```python
from build123d import *

# Parameters (mm, degrees)
EXTRUDE_1_DEPTH        = 196
CUT_EXTRUDE_1_DEPTH    = 240.62524927
SKETCH_4_W             = 106
SKETCH_4_H             = 19
CUT_EXTRUDE_2_DEPTH    = 242.065053461
SKETCH_6_W             = 106
SKETCH_6_H             = 129
CUT_EXTRUDE_3_DEPTH    = 242.065053461
SKETCH_7_W             = 20
SKETCH_7_H             = 5
EXTRUDE_3_DEPTH        = 15
PATTERN_LINEAR_1_COUNT = 2
PATTERN_LINEAR_1_PITCH = 60
CUT_EXTRUDE_6_REACH    = 244.147
SKETCH_10_W            = 182
SKETCH_10_H            = 30.218365382
CUT_EXTRUDE_7_REACH    = 254.973
SKETCH_12_W            = 180
SKETCH_12_H            = 40.166727714
CUT_EXTRUDE_8_REACH    = 254.973
SKETCH_13_W            = 129
SKETCH_13_H            = 8
SKETCH_14_W            = 20
SKETCH_14_H            = 5
EXTRUDE_4_DEPTH        = 15
PATTERN_LINEAR_2_COUNT = 2
PATTERN_LINEAR_2_PITCH = 60
FILLET_1_R             = 2
FILLET_2_R             = 2
FILLET_3_R             = 2
FILLET_4_R             = 2


with BuildPart() as part:
    # 草图1 → 凸台-拉伸1 (new body)
    with BuildSketch(Plane.XY):
        Polygon((0, 0), (-23, 0), (-23, 16.4), (2, 16.4), (2, 22.4), (-30, 22.4), (-30, -69.593534811), (-25.456561805, -69.593534811), (-9.398235911, -60), (119, -60), (119, -35), (114, -35), (114, -52), (0, -52), align=None)
    extrude(amount=EXTRUDE_1_DEPTH)

    # 草图2 → 切除-拉伸1 (cut, through all)
    with BuildSketch(Plane.XY.offset(196)):
        Polygon((-25, -5), (-25, -61.166727714), (-5, -49.218365382), (-5, -5), align=None)
    extrude(amount=-CUT_EXTRUDE_1_DEPTH, mode=Mode.SUBTRACT)

    # 草图4 → 切除-拉伸2 (cut, through all)
    with BuildSketch(Plane(origin=(0, -52, 0), x_dir=(1, 0, 0), z_dir=(0, 1, 0))):
        with Locations((61, -32.5)):
            Rectangle(SKETCH_4_W, SKETCH_4_H)
    extrude(amount=-CUT_EXTRUDE_2_DEPTH, mode=Mode.SUBTRACT)

    # 草图6 → 切除-拉伸3 (cut, through all)
    with BuildSketch(Plane(origin=(0, -52, 0), x_dir=(1, 0, 0), z_dir=(0, 1, 0))):
        with Locations((61, -116.5)):
            Rectangle(SKETCH_6_W, SKETCH_6_H)
    extrude(amount=-CUT_EXTRUDE_3_DEPTH, mode=Mode.SUBTRACT)

    # 草图7 → 凸台-拉伸3 (add)
    with BuildSketch(Plane(origin=(0, -52, 0), x_dir=(1, 0, 0), z_dir=(0, 1, 0))):
        with Locations((33, -193.5)):
            Rectangle(SKETCH_7_W, SKETCH_7_H)
    extrude_3 = extrude(amount=EXTRUDE_3_DEPTH)

    # 阵列(线性)1: 凸台-拉伸3 ×2
    with Locations(*[(i * PATTERN_LINEAR_1_PITCH, 0, 0) for i in range(1, PATTERN_LINEAR_1_COUNT)]):
        add(extrude_3)

    # 草图10 → 切除-拉伸6 (cut, up to next)
    with BuildSketch(Plane.ZY.offset(5), mode=Mode.PRIVATE) as cut_extrude_6_sk1:
        with Locations((98, -27.109182691)):
            Rectangle(SKETCH_10_W, SKETCH_10_H)
    cut_extrude_6_tool1 = extrude(cut_extrude_6_sk1.sketch, amount=-CUT_EXTRUDE_6_REACH, mode=Mode.PRIVATE) & part.part
    add(cut_extrude_6_tool1.solids().sort_by_distance((-5, -27.109183, 98))[0], mode=Mode.SUBTRACT)

    # 草图12 → 切除-拉伸7 (cut, up to next)
    with BuildSketch(Plane(origin=(-25, 0, 0), x_dir=(0, 0, -1), z_dir=(1, 0, 0)), mode=Mode.PRIVATE) as cut_extrude_7_sk1:
        with Locations((-98, -33.083363857)):
            Rectangle(SKETCH_12_W, SKETCH_12_H)
    cut_extrude_7_tool1 = extrude(cut_extrude_7_sk1.sketch, amount=-CUT_EXTRUDE_7_REACH, mode=Mode.PRIVATE) & part.part
    add(cut_extrude_7_tool1.solids().sort_by_distance((-25, -33.083364, 98))[0], mode=Mode.SUBTRACT)

    # 草图13 → 切除-拉伸8 (cut, up to next)
    with BuildSketch(Plane.ZY.offset(-114), mode=Mode.PRIVATE) as cut_extrude_8_sk1:
        with Locations((116.5, -56)):
            Rectangle(SKETCH_13_W, SKETCH_13_H)
    cut_extrude_8_tool1 = extrude(cut_extrude_8_sk1.sketch, amount=-CUT_EXTRUDE_8_REACH, mode=Mode.PRIVATE) & part.part
    add(cut_extrude_8_tool1.solids().sort_by_distance((114, -56, 116.5))[0], mode=Mode.SUBTRACT)

    # 草图14 → 凸台-拉伸4 (add)
    with BuildSketch(Plane(origin=(0, -52, 0), x_dir=(1, 0, 0), z_dir=(0, 1, 0))):
        with Locations((33, -2.5)):
            Rectangle(SKETCH_14_W, SKETCH_14_H)
    extrude_4 = extrude(amount=EXTRUDE_4_DEPTH)

    # 阵列(线性)2: 凸台-拉伸4 ×2
    with Locations(*[(i * PATTERN_LINEAR_2_PITCH, 0, 0) for i in range(1, PATTERN_LINEAR_2_COUNT)]):
        add(extrude_4)

    # 圆角1
    fillet_1_edges = [part.edges().sort_by_distance(p)[0] for p in [
        (2, 19.4, 0),
        (-14, 22.4, 0),
        (2, 22.4, 98),
        (-30, 22.4, 98),
        (-14, 22.4, 196),
        (2, 19.4, 196),
    ]]
    fillet(fillet_1_edges, radius=FILLET_1_R)

    # 圆角2
    fillet_2_edges = [part.edges().sort_by_distance(p)[0] for p in [
        (119, -60, 26),
        (119, -47.5, 0),
        (54.800882044, -60, 0),
        (54.800882044, -60, 196),
        (119, -60, 188.5),
        (119, -47.5, 196),
    ]]
    fillet(fillet_2_edges, radius=FILLET_2_R)

    # 圆角3
    fillet_3_edges = [part.edges().sort_by_distance(p)[0] for p in [
        (119, -52, 116.5),
        (115.5, -35, 196),
        (115.5, -35, 0),
        (119, -35, 98),
        (118.414213562, -35, 0.585786438),
        (118.414213562, -35, 195.414213562),
    ]]
    fillet(fillet_3_edges, radius=FILLET_3_R)

    # 圆角4
    fillet_4_edges = [part.edges().sort_by_distance(p)[0] for p in [
        (62.5, -60, 52),
        (118.414213562, -59.414213562, 52),
        (62.5, -60, 181),
        (118.414213562, -59.414213562, 181),
        (119, -54, 52),
        (119, -54, 181),
    ]]
    fillet(fillet_4_edges, radius=FILLET_4_R - 0.0001)  # a hair under: the kernel refuses the full size


solid = part.part
```
Input: part model. Units: mm. Frame: model coordinates. A direction names the side the tool comes from. Round coordinates to 2 decimals unless told otherwise and drop trailing zeros. Loops run counter-clockwise (first coordinate to the right, second up) from the corner with the lowest first, then second, coordinate; pieces in that order, holes last. Notation, with made-up numbers: M -5,59 L 41,59 A25 ccw 41,71 Z; hole C -33,15.5 d11. An arc over 180 degrees is marked long. Answer in a Markdown table with one row per item. Add a question column.
1. Section D-D (x = 99). Output: boundary loops of the cut face in (y, z).
2. Section A-A (x = 59.5). Output: boundary loops of the cut face in (y, z).
3. Contact query for flat-ended pins moving along their axis: pin 1 (1.5 mm diameter, centred on y = -56.5, z = 106, fed in from +X); pin 2 (1.5 mm diameter, centred on x = 115, z = 88.5, fed in from -Y); pin 3 (6 mm diameter, centred on y = -13.5, z = 104, fed in from +X). Output: stop coordinate, or through.
4. Mould query, pull axis Z, two halves, no side actions, for faces 6 (the face through (8, -56, 33)), 7 (the face through (27, -38, 196)), 8 (the face through (27, -38, 0)). Classes: released by +Z, released by -Z, zero draft, split by the parting line, or undercut.
5. Ray query, probe 1 along Y at (x, z) = (-1, 46); probe 2 along Z at (x, y) = (40, -53); probe 3 along Y at (x, z) = (-12.5, 50). Return the intervals inside material, ascending.
6. Set-up query: faces 1 (the face through (-27, -13, 99)), 2 (the face through (-15, -5, 99)), 3 (the face through (2, 18, 97)), 4 (the face through (-11, 16.4, 97)), 5 (the face through (23, -45, 194)). Return all of +Z, -Z, +X, -X, +Y, -Y with unobstructed straight access to the full face (end or side cutting, diameter ignored); none if empty.
7. Section C-C (z = 138.5). Give the number of separate pieces and of enclosed holes in the cut face, and give its area (3 significant figures).
8. Section B-B (y = -16). Output: boundary loops of the cut face in (x, z), and give its area (3 significant figures).
Values follow:
| question | item | result |
|---|---|---|
| 1 | outline | M -60,2 A2 ccw -58,0 L -37,0 L -37,5 L -52,5 L -52,23 L -60,23 Z; M -60,42 L -52,42 L -52,52 L -58,52 A2 ccw -60,50 Z; M -60,183 A2 ccw -58,181 L -52,181 L -52,191 L -37,191 L -37,196 L -58,196 A2 ccw -60,194 Z |
| 2 | outline | M -60,2 A2 ccw -58,0 L -52,0 L -52,23 L -60,23 Z; M -60,42 L -52,42 L -52,52 L -58,52 A2 ccw -60,50 Z; M -60,183 A2 ccw -58,181 L -52,181 L -52,196 L -58,196 A2 ccw -60,194 Z |
| 3 | pin 1 | x = 8 |
| 3 | pin 2 | y = -52 |
| 3 | pin 3 | x = 0 |
| 4 | face 6 | undercut |
| 4 | face 7 | released by +Z |
| 4 | face 8 | released by -Z |
| 5 | probe 1 | -60 to -42.22, -12 to 0, 16.4 to 22.4 |
| 5 | probe 2 | 0 to 23, 42 to 52, 181 to 196 |
| 5 | probe 3 | -61.85 to -53.7, -5 to 0, 16.4 to 22.4 |
| 6 | face 1 | +X, -X |
| 6 | face 2 | +Z, -Z |
| 6 | face 3 | +Z, -Z, +X, +Y |
| 6 | face 4 | +Z, -Z, +X |
| 6 | face 5 | +Z, -Z, +Y |
| 7 | separate pieces | 3 |
| 7 | enclosed holes | 0 |
| 7 | area | 1,020 mm^2 |
| 8 | outline | M -30,0 L -25,0 L -25,8 L -30,8 Z; M -30,188 L -25,188 L -25,196 L -30,196 Z; M -5,0 L 0,0 L 0,7 L -5,7 Z; M -5,189 L 0,189 L 0,196 L -5,196 Z |
| 8 | area | 150 mm^2 |
